Work out the finished part from the listing and answer in its coordinate system (mm). A direction names the side the tool comes from. Give positions to 0.01 mm unless a question says otherwise; leave off trailing zeros. Order: outer loops, then holes, each group sorted by start corner. A loop starts at its lowest first (then second) coordinate and runs counter-clockwise, first axis right, second up. Notation, with made-up numbers: (43, -2) - (78, -2) arc R24 cw to (78, 31) - close; hole circle Ø8 at (50.25, 27). An arc over 180 degrees is marked (long way). Put each result on its own line as item: value.
```python
from build123d import *

# Parameters (mm, degrees)
F0_W     = 30.374784
F0_H     = 50.35834
F0_W_2   = 25.623474
F0_H_2   = 49.36993
F0_W_3   = 4.138445
F0_H_3   = 1.773622
F1_DEPTH = 10.414
F2_SIZE  = 5.08


with BuildPart() as f1:
    # F0 (on Top) → F1 (new body)
    with BuildSketch(Plane.XY):
        Polygon((-30.374784, 24.338016), (-36.359224, 24.338016), (-36.359224, 14.719548), (-36.359224, -38.724054), (0, -38.724054), (0, -26.020324), (-30.374784, -26.020324), align=None)
        Polygon((-36.359224, 14.719548), (-36.359224, 24.338016), (-86.168446, 24.338016), (-86.168446, 14.719548), (-77.702753, 14.719548), (-52.079279, 14.719548), align=None)
        with Locations((-15.187392, -0.841154)):
            Rectangle(F0_W, F0_H)
        Polygon((22.958538, 24.338016), (0, 24.338016), (0, -26.020324), (0, -38.724054), (27.096983, -38.724054), (27.096983, 24.338016), align=None)
        with Locations((-64.891016, -9.965417)):
            Rectangle(F0_W_2, F0_H_2)
        with Locations((25.02776, 25.224827)):
            Rectangle(F0_W_3, F0_H_3)
        Polygon((27.096983, -38.724054), (0, -38.724054), (0, -62.185474), (90.715356, -62.185474), (90.715356, 24.338016), (27.096983, 24.338016), align=None)
    extrude(amount=F1_DEPTH)

    # F2
    f2_edges = [f1.edges().sort_by_distance(p)[0] for p in [
        (-86.168446, 24.338016, 5.207),
        (-36.359224, -38.724054, 5.207),
        (90.715356, 24.338016, 5.207),
    ]]
    chamfer(f2_edges, length=F2_SIZE)


solid = f1.part
```
(1) Section B-B, the plane z = 4.25 is taken. Write down the section's boundary in (x, y), then the cut area to 3 significant figures.
Geometry check:
outline: (-86.17, 14.72) - (-77.7, 14.72) - (-77.7, -34.65) - (-52.08, -34.65) - (-52.08, 14.72) - (-36.36, 14.72) - (-36.36, -33.64) - (-31.28, -38.72) - (0, -38.72) - (0, -62.19) - (90.72, -62.19) - (90.72, 19.26) - (85.64, 24.34) - (27.1, 24.34) - (27.1, 26.11) - (22.96, 26.11) - (22.96, 24.34) - (-81.09, 24.34) - (-86.17, 19.26) - close
area: 11,900 mm²
(2) Straight lines are drawn through the part: line 1 (X direction, y = -3.5, z = 7); line 2 (X direction, y = -58, z = 5); line 3 (Y direction, x = 3.5, z = 7.5). For each, find the intervals that lie inside material, in ascending order.
Geometry check:
line 1: x = -77.7 to -52.08, -36.36 to 90.72
line 2: x = 0 to 90.72
line 3: y = -62.19 to 24.34
(3) A tool of negligible diameter and unlimited length cuts with its end or side. For faces 1 (the face through (-16, -38.724, 5)), 2 (the face through (-44, 14.72, 5)), 3 (the face through (-28, 24.338, 5)), from which of +Z, -Z, +X, -X, +Y, -Y can it reach the whole face along a straight path? Write none if from no direction.
Geometry check:
face 1: +Z, -Z, -X, -Y
face 2: +Z, -Z, -Y
face 3: +Z, -Z, -X, +Y
(4) Determine the mould class of faces 4 (the face through (25, 26.112, 5)), 5 (the face through (90.715, -22, 5)), 6 (the face through (-36.359, -9, 5)) for opening direction X: pulls with the +X half, pulls with the -X half, needs draft (parallel to the pull), parting line crosses it, or undercut.
Geometry check:
face 4: needs draft
face 5: pulls with the +X half
face 6: undercut
(5) Section D-D, the plane y = -42 is taken. Write down the section's boundary in (x, z).
Geometry check:
outline: (0, 0) - (90.72, 0) - (90.72, 10.41) - (0, 10.41) - close
(6) Section C-C, the plane x = -39 is taken. Write down the section's boundary in (y, z).
Geometry check:
outline: (14.72, 0) - (24.34, 0) - (24.34, 10.41) - (14.72, 10.41) - close
(7) Section A-A, the plane y = -2 is taken. Write down the section's boundary in (x, z).
Geometry check:
outline: (-77.7, 0) - (-52.08, 0) - (-52.08, 10.41) - (-77.7, 10.41) - close; (-36.36, 0) - (90.72, 0) - (90.72, 10.41) - (-36.36, 10.41) - close
(8) Given pin 1 (6 mm diameter, centred on y = -45, z = 2, fed in from -X); pin 2 (1 mm diameter, centred on x = -19, z = 2.5, fed in from -Y); pin 3 (1.5 mm diameter, centred on x = -62, z = 2, fed in from +Y), each flat-ended and moving along its own axis, determine where each tip first touches the part or whether it passes through.
Geometry check:
pin 1: stops at x = 0
pin 2: stops at y = -38.72
pin 3: stops at y = 24.34
